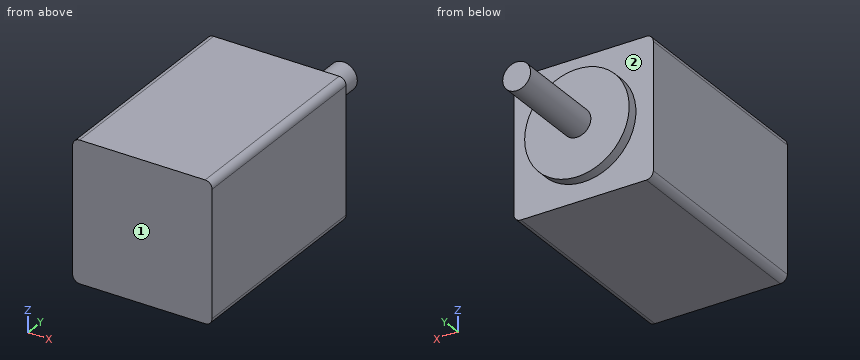
from build123d import *

# Parameters (mm, degrees)
F0_W     = 20
F0_H     = 20
F0_R     = 7.5
F0_R_2   = 2
F1_DEPTH = 30
F2_DEPTH = 15
F3_R     = 1
F4_DEPTH = 1.5


with BuildPart() as f1:
    # F0 (on Front) → F1 (new body)
    with BuildSketch(Plane.XZ):
        Rectangle(F0_W, F0_H)
        Circle(F0_R, mode=Mode.SUBTRACT)
        Circle(F0_R)
        Circle(F0_R_2, mode=Mode.SUBTRACT)
        Circle(F0_R_2)
    extrude(amount=F1_DEPTH)

    # F0 (on Front) → F2 (join)
    with BuildSketch(Plane.XZ):
        Circle(F0_R_2)
    extrude(amount=-F2_DEPTH)

    # F3
    f3_edges = [f1.edges().sort_by_distance(p)[0] for p in [
        (10, -15, 10),
        (-10, -15, 10),
        (-10, -15, -10),
        (10, -15, -10),
    ]]
    fillet(f3_edges, radius=F3_R)

    # F0 (on Front) → F4 (join)
    with BuildSketch(Plane.XZ):
        Circle(F0_R)
        Circle(F0_R_2, mode=Mode.SUBTRACT)
    extrude(amount=-F4_DEPTH)


solid = f1.part
Verification items for the finished model (mm, model axes). Face numbers are marked on the shaded views. A direction names the side the tool comes from. Give positions to 0.01 mm unless a question says otherwise; leave off trailing zeros. Loops run counter-clockwise (first coordinate to the right, second up) from the corner with the lowest first, then second, coordinate; pieces in that order, holes last.
1) Sectioned sample at A-A, the plane x = 0. Enter the section's corners in (y, z), then the cut area to 4 significant figures.
2) Sectioned sample at C-C, the plane y = 7. Enter the section's corners in (x, z).
3) Depth check by flat-ended pin: pin 1 Ø6 at (x, z) = (-4, -4) entering from +Y; pin 2 Ø6 at (y, z) = (4, 4.5) entering from -X. Enter the tip coordinate at first touch or a pass-through.
4) Set-up check for the marked faces 1 and 2: record each of +Z, -Z, +X, -X, +Y, -Y from which the full face is reachable in a straight line by a thin tool's end or side.
5) Thickness scan on line 1 along Y through (x, z) = (3.25, -2.25); line 2 along Y through (x, z) = (-8.75, 2.25); line 3 along X through (y, z) = (1, -0.5). Record the ranges inside material, lowest first.
6) Sectioned sample at B-B, the plane z = 0. Enter the section's corners in (x, y).
7) Sectioned sample at D-D, the plane x = 2.75. Enter the section's corners in (y, z), then the cut area to 3 significant figures.
Answers:
1. outline: (-30, -10) - (0, -10) - (0, -7.5) - (1.5, -7.5) - (1.5, -2) - (15, -2) - (15, 2) - (1.5, 2) - (1.5, 7.5) - (0, 7.5) - (0, 10) - (-30, 10) - close
1. area: 676.5 mm2
2. outline: circle Ø4 at (0, 0)
3. pin 1: stops at y = 1.5
3. pin 2: stops at x = -6.94
4. face 1: +Z, -Z, +X, -X, -Y
4. face 2: +Y
5. line 1: y = -30 to 1.5
5. line 2: y = -30 to 0
5. line 3: x = -7.48 to 7.48
6. outline: (-10, -30) - (10, -30) - (10, 0) - (7.5, 0) - (7.5, 1.5) - (2, 1.5) - (2, 15) - (-2, 15) - (-2, 1.5) - (-7.5, 1.5) - (-7.5, 0) - (-10, 0) - close
7. outline: (-30, -10) - (0, -10) - (0, -6.98) - (1.5, -6.98) - (1.5, 6.98) - (0, 6.98) - (0, 10) - (-30, 10) - close
7. area: 621 mm2
